Design review of the part shown in the three views and the two pictorial views. Dimensions are in mm from the part's minimum x, y and z. A direction names the side the tool comes from. Coordinates: 2 decimals unless noted, no trailing zeros. Loops run counter-clockwise (first coordinate to the right, second up) from the corner with the lowest first, then second, coordinate; pieces in that order, holes last.
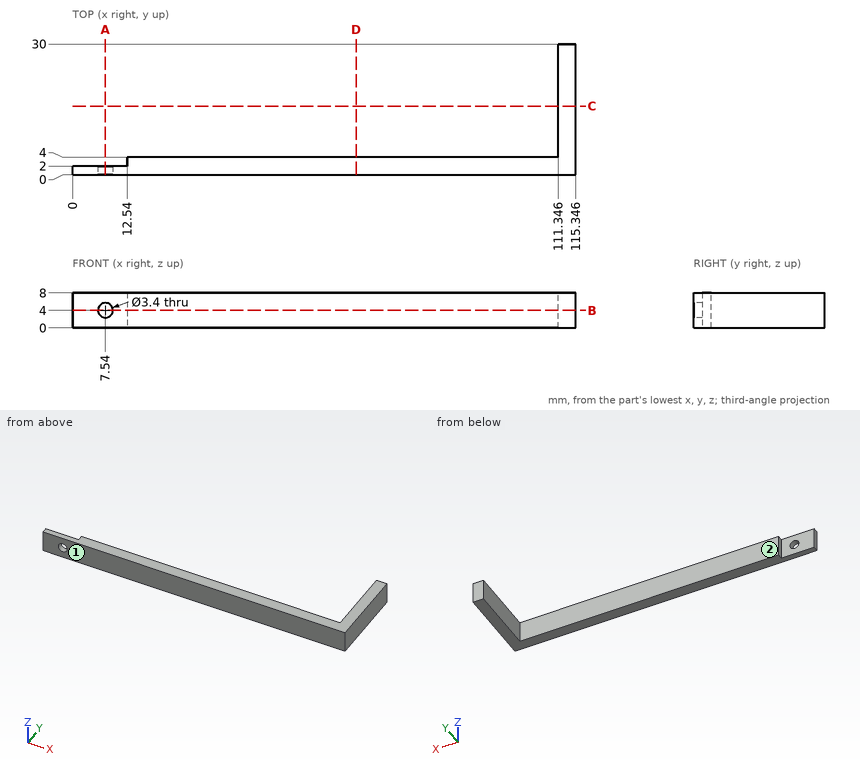
Q1. Consider section B-B (z = 4). State the section outline as (x, y) points.
Q2. Machinability: for the marked faces 1 and 2, which of the approach directions +Z, -Z, +X, -X, +Y, -Y give a long, thin tool a straight path to every point of the face, cutting with its end or side? Answer none if there is none.
Q3. Consider section A-A (x = 7.54). State the section outline as (y, z) points.
Q4. Consider section D-D (x = 65). State the section outline as (y, z) points.
Q5. Consider section C-C (y = 15.75). State the section outline as (x, z) points.
Q6. Wall thickness on probe 1 along X at (y, z) = (0.5, 4); probe 2 along X at (y, z) = (5.75, 3.5); probe 3 along Y at (x, z) = (78.5, 5.75): over which ranges is each line inside the solid? List them lowest first.
Q7. For pin 1 Ø4 at (x, z) = (9, 5) entering from +Y; pin 2 Ø4 at (x, z) = (68.5, 6) entering from +Y; pin 3 Ø4 at (y, z) = (12, 5) entering from -X, all flat-tipped, find the tip position at first contact; note any pin that passes through.
Model answer:
1. outline: (0, 0) - (5.84, 0) - (5.84, 2) - (0, 2) - close; (9.24, 0) - (115.35, 0) - (115.35, 30) - (111.35, 30) - (111.35, 4) - (12.54, 4) - (12.54, 2) - (9.24, 2) - close
2. face 1: +Z, -Z, +X, -X, -Y
2. face 2: +Z, -Z, -X, +Y
3. outline: (0, 0) - (2, 0) - (2, 2.3) - (0, 2.3) - close; (0, 5.7) - (2, 5.7) - (2, 8) - (0, 8) - close
4. outline: (0, 0) - (4, 0) - (4, 8) - (0, 8) - close
5. outline: (111.35, 0) - (115.35, 0) - (115.35, 8) - (111.35, 8) - close
6. probe 1: x = 0 to 5.84, 9.24 to 115.35
6. probe 2: x = 111.35 to 115.35
6. probe 3: y = 0 to 4
7. pin 1: stops at y = 2
7. pin 2: stops at y = 4
7. pin 3: stops at x = 111.35
